Build history of the part. All positions in model axes, mm. Face numbers are marked on the shaded views. A direction names the side the tool comes from. Coordinates: 2 decimals unless noted, no trailing zeros. Order: outer loops, then holes, each group sorted by start corner. A loop starts at its lowest first (then second) coordinate and runs counter-clockwise, first axis right, second up. Notation, with made-up numbers: (28.25, 25.5) - (72.25, 25.5) arc R27 cw to (72.25, 63.5) - close; hole circle Ø3 at (64.25, 64). An arc over 180 degrees is marked (long way). Return JSON: item names as keys, results as strings.
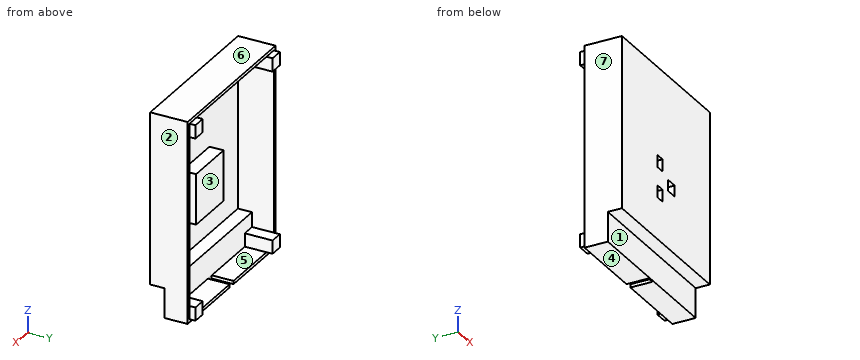
from build123d import *

# Parameters (mm, degrees)
SKETCH5_W           = 100
SKETCH5_H           = 11.6
BOSS_EXTRUDE3_DEPTH = 80
SKETCH6_W           = 85.25
SKETCH6_H           = 7
BOSS_EXTRUDE4_DEPTH = 80
SKETCH7_W           = 76.8
SKETCH7_H           = 96.8
CUT_EXTRUDE1_DEPTH  = 10.8
SKETCH8_W           = 76.8
SKETCH8_H           = 82.85
CUT_EXTRUDE2_DEPTH  = 7
SKETCH10_W          = 6.6
SKETCH10_H          = 6.6
BOSS_EXTRUDE5_DEPTH = 17.8
SKETCH12_W          = 6.6
SKETCH12_H          = 6.6
BOSS_EXTRUDE6_DEPTH = 10.8
SKETCH15_W          = 3.5
SKETCH15_H          = 10.858624792
CUT_EXTRUDE4_DEPTH  = 1.6
SKETCH16_W          = 6.6
SKETCH16_H          = 6.6
BOSS_EXTRUDE8_DEPTH = 3
SKETCH18_W          = 25
SKETCH18_H          = 25
BOSS_EXTRUDE9_DEPTH = 7
SKETCH19_W          = 4.5
SKETCH19_H          = 6
SKETCH19_W_2        = 6
SKETCH19_H_2        = 5.5
CUT_EXTRUDE5_DEPTH  = 6.2


with BuildPart() as part:
    # Sketch5 → Boss-Extrude3 (new body)
    with BuildSketch(Plane(origin=(0, 0, 0), x_dir=(0, 0, -1), z_dir=(1, 0, 0))):
        with Locations((50, 5.8)):
            Rectangle(SKETCH5_W, SKETCH5_H)
    extrude(amount=BOSS_EXTRUDE3_DEPTH)

    # Sketch7 → Cut-Extrude1 (cut)
    with BuildSketch(Plane(origin=(0, 11.6, 0), x_dir=(1, 0, 0), z_dir=(0, 1, 0))):
        with Locations((40, 50)):
            Rectangle(SKETCH7_W, SKETCH7_H)
    extrude(amount=-CUT_EXTRUDE1_DEPTH, mode=Mode.SUBTRACT)


with BuildPart() as body_2:
    # Sketch6 → Boss-Extrude4 (new body)
    with BuildSketch(Plane(origin=(80, 0, 0), x_dir=(0, 0, -1), z_dir=(1, 0, 0))):
        with Locations((42.625, -3.5)):
            Rectangle(SKETCH6_W, SKETCH6_H)
    extrude(amount=-BOSS_EXTRUDE4_DEPTH)


with BuildPart() as cut_extrude2_tool:
    # Sketch8 → Cut-Extrude2 (new body)
    with BuildSketch(Plane(origin=(0, 0.8, 0), x_dir=(1, 0, 0), z_dir=(0, 1, 0))):
        with Locations((40, 43.025)):
            Rectangle(SKETCH8_W, SKETCH8_H)
    extrude(amount=-CUT_EXTRUDE2_DEPTH)


with BuildPart() as part_1:
    add(part.part)

    # Cut-Extrude2: cut by cut_extrude2_tool
    add(cut_extrude2_tool.part, mode=Mode.SUBTRACT)



with BuildPart() as body_2_1:
    add(body_2.part)

    # Cut-Extrude2: cut by cut_extrude2_tool
    add(cut_extrude2_tool.part, mode=Mode.SUBTRACT)


with BuildPart() as part_2:
    add(part_1.part)

    add(body_2_1.part)  # Boss-Extrude5 merges body 2
    # Sketch10 → Boss-Extrude5 (add)
    with BuildSketch(Plane(origin=(0, -6.2, 0), x_dir=(1, 0, 0), z_dir=(0, 1, 0))):
        with Locations((4.9, 4.9)):
            Rectangle(SKETCH10_W, SKETCH10_H)
        with Locations((75.1, 4.9)):
            Rectangle(SKETCH10_W, SKETCH10_H)
    extrude(amount=BOSS_EXTRUDE5_DEPTH)

    # Sketch12 → Boss-Extrude6 (add)
    with BuildSketch(Plane(origin=(0, 0.8, 0), x_dir=(1, 0, 0), z_dir=(0, 1, 0))):
        with Locations((4.9, 95.1)):
            Rectangle(SKETCH12_W, SKETCH12_H)
        with Locations((75.1, 95.1)):
            Rectangle(SKETCH12_W, SKETCH12_H)
    extrude(amount=BOSS_EXTRUDE6_DEPTH)

    # Sketch15 → Cut-Extrude4 (cut)
    with BuildSketch(Plane(origin=(0, 0, -100), x_dir=(-1, 0, 0), z_dir=(0, 0, -1))):
        with Locations((-40, 6.170687604)):
            Rectangle(SKETCH15_W, SKETCH15_H)
    extrude(amount=-CUT_EXTRUDE4_DEPTH, mode=Mode.SUBTRACT)

    # Sketch16 → Boss-Extrude8 (add)
    with BuildSketch(Plane(origin=(0, 11.6, 0), x_dir=(1, 0, 0), z_dir=(0, 1, 0))):
        with Locations((4.9, 95.1)):
            Rectangle(SKETCH16_W, SKETCH16_H)
        with Locations((75.1, 4.9)):
            Rectangle(SKETCH16_W, SKETCH16_H)
        with Locations((4.9, 4.9)):
            Rectangle(SKETCH16_W, SKETCH16_H)
        with Locations((75.1, 95.1)):
            Rectangle(SKETCH16_W, SKETCH16_H)
    extrude(amount=BOSS_EXTRUDE8_DEPTH)

    # Sketch18 → Boss-Extrude9 (add)
    with BuildSketch(Plane(origin=(0, -6.2, 0), x_dir=(1, 0, 0), z_dir=(0, 1, 0))):
        with Locations((40, 54.1)):
            Rectangle(SKETCH18_W, SKETCH18_H)
    extrude(amount=BOSS_EXTRUDE9_DEPTH)

    # Sketch19 → Cut-Extrude5 (cut)
    with BuildSketch(Plane.XZ.offset(7)):
        with Locations((34.75, -46.6)):
            Rectangle(SKETCH19_W, SKETCH19_H)
        with Locations((34.75, -61.6)):
            Rectangle(SKETCH19_W, SKETCH19_H)
        with Locations((45, -54.1)):
            Rectangle(SKETCH19_W_2, SKETCH19_H_2)
    extrude(amount=-CUT_EXTRUDE5_DEPTH, mode=Mode.SUBTRACT)


solid = part_2.part
1. Mould opens along Z. For the marked faces 4, 5, 6 and 7 say: pulls with the +Z half, pulls with the -Z half, needs draft (parallel to the pull), parting line crosses it, or undercut.
Check values:
{"face 4": "pulls with the -Z half", "face 5": "undercut", "face 6": "pulls with the +Z half", "face 7": "needs draft"}
2. Drop flat-ended pins along their axis: pin 1 (2.5 mm diameter, centred on x = 75.5, y = 13, fed in from -Z); pin 2 (1.8 mm diameter, centred on x = 39, z = -99.5, fed in from +Y); pin 3 (12 mm diameter, centred on x = 53, z = -95, fed in from -Y). Give the stop position or say it passes through.
Check values:
{"pin 1": "z = -98.4", "pin 2": "y = 11.6", "pin 3": "y = 0"}
3. Cut at A-A on y = -3. Give the cut face in (x, z).
Check values:
{"outline": "(0, -85.25) - (80, -85.25) - (80, 0) - (0, 0) - close; (27.5, -66.6) - (52.5, -66.6) - (52.5, -41.6) - (27.5, -41.6) - close; hole (1.6, -84.45) - (78.4, -84.45) - (78.4, -8.2) - (71.8, -8.2) - (71.8, -1.6) - (8.2, -1.6) - (8.2, -8.2) - (1.6, -8.2) - close; hole (32.5, -64.6) - (37, -64.6) - (37, -58.6) - (32.5, -58.6) - close; hole (32.5, -49.6) - (37, -49.6) - (37, -43.6) - (32.5, -43.6) - close; hole (42, -56.85) - (48, -56.85) - (48, -51.35) - (42, -51.35) - close"}
4. Cut at D-D on z = -88. Give the cut face in (x, y).
Check values:
{"outline": "(0, 0) - (80, 0) - (80, 11.6) - (78.4, 11.6) - (78.4, 0.8) - (1.6, 0.8) - (1.6, 11.6) - (0, 11.6) - close"}
5. Cut at C-C on x = 16.5. Give the cut face in (y, z), plus the area to 3 significant figures.
Check values:
{"outline": "(-7, -85.25) - (0, -85.25) - (0, -100) - (11.6, -100) - (11.6, -98.4) - (0.8, -98.4) - (0.8, -84.45) - (-6.2, -84.45) - (-6.2, -1.6) - (11.6, -1.6) - (11.6, 0) - (-7, 0) - close", "area": "131 mm²"}
6. Tool access for the marked faces 1, 2 and 3: list every direction of +Z, -Z, +X, -X, +Y, -Y with a clear straight run to the whole face (end or side of a thin tool).
Check values:
{"face 1": "-Z, +X, -X, -Y", "face 2": "+Z, -Z, +X, +Y, -Y", "face 3": "+Y"}
7. Probe L1, parallel to Z at x = 51, y = -0.25; L2, parallel to Z at x = 4.5, y = 2.5; L3, parallel to X at y = 1.75, z = -67. List the from-to ranges inside material, lowest first.
Check values:
{"L1": "-85.25 to -84.45, -66.6 to -41.6, -1.6 to 0", "L2": "-100 to -91.8, -8.2 to 0", "L3": "0 to 1.6, 78.4 to 80"}
8. Cut at B-B on y = 7. Give the cut face in (x, z), plus the area to 3 significant figures.
Check values:
{"outline": "(0, -100) - (38.25, -100) - (38.25, -98.4) - (8.2, -98.4) - (8.2, -91.8) - (1.6, -91.8) - (1.6, -8.2) - (8.2, -8.2) - (8.2, -1.6) - (71.8, -1.6) - (71.8, -8.2) - (78.4, -8.2) - (78.4, -91.8) - (71.8, -91.8) - (71.8, -98.4) - (41.75, -98.4) - (41.75, -100) - (80, -100) - (80, 0) - (0, 0) - close", "area": "734 mm²"}
